For this review, take the finished solid that the model builds, in its own axes (mm). A direction names the side the tool comes from. Coordinates: 2 decimals unless noted, no trailing zeros. Loops run counter-clockwise (first coordinate to the right, second up) from the corner with the lowest first, then second, coordinate; pieces in that order, holes last. Notation, with made-up numbers: (22.5, -33.75) -> (37.5, -33.75) arc R36 cw to (37.5, 1.25) -> close; hole circle Ø4 at (11, 49). An arc over 180 degrees is marked (long way). One line per item, written item: value.
from build123d import *

# Parameters (mm, degrees)
SKETCH1_R                               = 55
BOSS_EXTRUDE1_DEPTH                     = 20
SKETCH2_R                               = 27.5
BOSS_EXTRUDE2_DEPTH                     = 30
SKETCH6_R                               = 23.5
CUT_EXTRUDE1_DEPTH                      = 15
FILLET1_R                               = 5
CBORE_FOR_M8_HEX_HEAD_BOLT1_D           = 9
CBORE_FOR_M8_HEX_HEAD_BOLT1_CBORE_D     = 18.011
CBORE_FOR_M8_HEX_HEAD_BOLT1_CBORE_DEPTH = 5.3
FILLET2_R                               = 4
SKETCH10_R                              = 13.5
CUT_EXTRUDE2_DEPTH                      = 53
SKETCH11_R                              = 22.5
SKETCH11_R_2                            = 13.5
BOSS_EXTRUDE3_DEPTH                     = 15
FILLET3_R                               = 5


with BuildPart() as part:
    # Sketch1 → Boss-Extrude1 (new body)
    with BuildSketch(Plane(origin=(0, 0, 0), x_dir=(1, 0, 0), z_dir=(0, 1, 0))):
        with Locations(Location((0, 0, 0), (0, 0, 270))):
            Circle(SKETCH1_R)
    extrude(amount=BOSS_EXTRUDE1_DEPTH)

    # Sketch2 → Boss-Extrude2 (add)
    with BuildSketch(Plane(origin=(0, 20, 0), x_dir=(1, 0, 0), z_dir=(0, 1, 0))):
        with Locations(Location((0, 0, 0), (0, 0, 270))):
            Circle(SKETCH2_R)
    extrude(amount=BOSS_EXTRUDE2_DEPTH)

    # Sketch6 → Cut-Extrude1 (cut)
    with BuildSketch(Plane(origin=(0, 50, 0), x_dir=(1, 0, 0), z_dir=(0, 1, 0))):
        with Locations(Location((0, 0, 0), (0, 0, 270))):
            Circle(SKETCH6_R)
    extrude(amount=-CUT_EXTRUDE1_DEPTH, mode=Mode.SUBTRACT)

    # Fillet1
    fillet1_edges = [part.edges().sort_by_distance(p)[0] for p in [
        (0, 20, -27.5),
    ]]
    fillet(fillet1_edges, radius=FILLET1_R)

    # CBORE for M8 Hex Head Bolt1 (through all)
    with Locations(Plane(origin=(-27.5, 0, 27.5), x_dir=(0, 0, -1), z_dir=(0, -1, 0))):
        with Locations((0, 0), (0, 55), (55, 55), (55, 0)):
            CounterBoreHole(CBORE_FOR_M8_HEX_HEAD_BOLT1_D / 2, CBORE_FOR_M8_HEX_HEAD_BOLT1_CBORE_D / 2, CBORE_FOR_M8_HEX_HEAD_BOLT1_CBORE_DEPTH)

    # Fillet2
    fillet2_edges = [part.edges().sort_by_distance(p)[0] for p in [
        (0, 0, -55),
    ]]
    fillet(fillet2_edges, radius=FILLET2_R)

    # Sketch10 → Cut-Extrude2 (cut)
    with BuildSketch(Plane(origin=(0, 35, 0), x_dir=(1, 0, 0), z_dir=(0, 1, 0))):
        with Locations(Location((0, 0, 0), (0, 0, 270))):
            Circle(SKETCH10_R)
    extrude(amount=-CUT_EXTRUDE2_DEPTH, mode=Mode.SUBTRACT)

    # Sketch11 → Boss-Extrude3 (add)
    with BuildSketch(Plane.XZ):
        with Locations(Location((0, 0, 0), (0, 0, 90))):
            Circle(SKETCH11_R)
        with Locations(Location((0, 0, 0), (0, 0, 90))):
            Circle(SKETCH11_R_2, mode=Mode.SUBTRACT)
    extrude(amount=BOSS_EXTRUDE3_DEPTH)

    # Fillet3
    fillet3_edges = [part.edges().sort_by_distance(p)[0] for p in [
        (0, 0, -22.5),
        (0, -15, -22.5),
    ]]
    fillet(fillet3_edges, radius=FILLET3_R)


solid = part.part
1. Insertion check: pin 1 Ø1.5 at (y, z) = (2, -41) entering from +X; pin 2 Ø14.5 at (x, z) = (-27.5, 27.5) entering from +Y; pin 3 Ø12 at (x, z) = (-6, -25) entering from -Y. Each pin has a flat end and moves straight along its axis. Give the tip position at first contact, or say it passes through.
Return value:
pin 1: stops at x = 36.86
pin 2: stops at y = 20.07
pin 3: stops at y = -14.49
2. For faces 4 (the cylindrical face through (13.18, 10.35, -2.93)), 5 (the cylindrical face through (15.88, 42.6, -17.32)), 6 (the flat face through (-29, 5.3, -23)), list the 3-axis set-ups (+Z, -Z, +X, -X, +Y, -Y) from which the entire face can be reached by the end or side of a thin tool; tool diameter is ignored.
Return value:
face 4: +Y, -Y
face 5: +Y
face 6: -Y
3. Take a section at C-C, the plane y = 9. Give the boundary of the cut face in (x, z), and give its area (3 significant figures).
Return value:
outline: circle Ø110 at (0, 0); hole circle Ø9 at (-27.5, -27.5); hole circle Ø9 at (-27.5, 27.5); hole circle Ø27 at (0, 0); hole circle Ø9 at (27.5, -27.5); hole circle Ø9 at (27.5, 27.5)
area: 8,680 mm2
4. Take a section at B-B, the plane z = 0. Give the boundary of the cut face in (x, y), and give its area (3 significant figures).
Return value:
outline: (-55, 4) arc R4 ccw to (-51, 0) -> (-27.5, 0) arc R5 cw to (-22.5, -5) -> (-22.5, -10) arc R5 ccw to (-17.5, -15) -> (-13.5, -15) -> (-13.5, 35) -> (-23.5, 35) -> (-23.5, 50) -> (-27.5, 50) -> (-27.5, 25) arc R5 cw to (-32.5, 20) -> (-55, 20) -> close; (13.5, -15) -> (17.5, -15) arc R5 ccw to (22.5, -10) -> (22.5, -5) arc R5 cw to (27.5, 0) -> (51, 0) arc R4 ccw to (55, 4) -> (55, 20) -> (32.5, 20) arc R5 cw to (27.5, 25) -> (27.5, 50) -> (23.5, 50) -> (23.5, 35) -> (13.5, 35) -> close
area: 2,470 mm2
5. The part is to be moulded in two halves that separate along X. For faces 1 (the cylindrical face through (18.71, 2.61, -25.55)), 2 (the cylindrical face through (8.618, -7.465, 20.784)), 3 (the flat face through (-33, 0, -1)), say which applies: pulls with the +X half, pulls with the -X half, needs draft (parallel to the pull), parting line crosses it, or undercut.
Return value:
face 1: undercut
face 2: parting line crosses it
face 3: needs draft
6. To check wall thickness, follow probe 1 along Z at (x, y) = (27, 1); probe 2 along X at (y, z) = (6.5, 0); probe 3 along X at (y, z) = (16, 27). State the ranges of each line that lie inside material, in increasing order. Write a range as from..to.
Return value:
probe 1: z = -46.36..-36.49, -18.51..18.51, 36.49..46.36
probe 2: x = -55..-13.5, 13.5..55
probe 3: x = -47.92..-31.97, -23.03..23.03, 31.97..47.92
7. Take a section at D-D, the plane y = 2.5. Give the boundary of the cut face in (x, z), and give its area (3 significant figures).
Return value:
outline: circle Ø109.42 at (0, 0); hole circle Ø18.01 at (-27.5, -27.5); hole circle Ø18.01 at (-27.5, 27.5); hole circle Ø27 at (0, 0); hole circle Ø18.01 at (27.5, -27.5); hole circle Ø18.01 at (27.5, 27.5)
area: 7,810 mm2
8. Take a section at A-A, the plane x = 0. Give the boundary of the cut face in (y, z), and give its area (3 significant figures).
Return value:
outline: (-15, -17.5) arc R5 ccw to (-10, -22.5) -> (-5, -22.5) arc R5 cw to (0, -27.5) -> (0, -51) arc R4 ccw to (4, -55) -> (20, -55) -> (20, -32.5) arc R5 cw to (25, -27.5) -> (50, -27.5) -> (50, -23.5) -> (35, -23.5) -> (35, -13.5) -> (-15, -13.5) -> close; (-15, 13.5) -> (35, 13.5) -> (35, 23.5) -> (50, 23.5) -> (50, 27.5) -> (25, 27.5) arc R5 cw to (20, 32.5) -> (20, 55) -> (4, 55) arc R4 ccw to (0, 51) -> (0, 27.5) arc R5 cw to (-5, 22.5) -> (-10, 22.5) arc R5 ccw to (-15, 17.5) -> close
area: 2,470 mm2
